```python
from build123d import *

# Parameters (mm, degrees)
EXTRUDE_1_DEPTH     = 3
FILLET_1_R          = 6
FILLET_2_R          = 2
SKETCH_2_R          = 1.65
CUT_EXTRUDE_1_DEPTH = 5
FILLET_3_R          = 10
SKETCH_3_W          = 90
SKETCH_3_H          = 4
CUT_EXTRUDE_2_DEPTH = 10
FILLET_4_R          = 10


with BuildPart() as part:
    # 草图1 → 凸台-拉伸1 (new body)
    with BuildSketch(Plane.XY):
        Polygon((25, 25), (45, 25), (45, -25), (-45, -25), (-45, 25), (-25, 25), (-25, 20), (-36, 20), (-36, 5), (36, 5), (36, 20), (25, 20), align=None)
    extrude(amount=EXTRUDE_1_DEPTH)

    # 圆角1
    fillet_1_edges = [part.edges().sort_by_distance(p)[0] for p in [
        (-45, 25, 1.5),
        (45, 25, 1.5),
    ]]
    fillet(fillet_1_edges, radius=FILLET_1_R)

    # 圆角2
    fillet_2_edges = [part.edges().sort_by_distance(p)[0] for p in [
        (-25, 25, 1.5),
        (-25, 20, 1.5),
        (-36, 20, 1.5),
        (-36, 5, 1.5),
        (36, 5, 1.5),
        (36, 20, 1.5),
        (25, 20, 1.5),
        (25, 25, 1.5),
    ]]
    fillet(fillet_2_edges, radius=FILLET_2_R)

    # 草图2 → 切除-拉伸1 (cut)
    with BuildSketch(Plane.XY.offset(3)):
        with Locations((-25, -10)):
            Circle(SKETCH_2_R)
        with Locations((25, -10)):
            Circle(SKETCH_2_R)
        with Locations((0, -10)):
            Circle(SKETCH_2_R)
    extrude(amount=-CUT_EXTRUDE_1_DEPTH, mode=Mode.SUBTRACT)

    # 圆角3
    fillet_3_edges = [part.edges().sort_by_distance(p)[0] for p in [
        (45, -25, 1.5),
        (-45, -25, 1.5),
    ]]
    fillet(fillet_3_edges, radius=FILLET_3_R)

    # 草图3 → 切除-拉伸2 (cut)
    with BuildSketch(Plane.XY.offset(3)):
        with Locations((0, -23)):
            Rectangle(SKETCH_3_W, SKETCH_3_H)
    extrude(amount=-CUT_EXTRUDE_2_DEPTH, mode=Mode.SUBTRACT)

    # 圆角4
    fillet_4_edges = [part.edges().sort_by_distance(p)[0] for p in [
        (43, -21, 1.5),
    ]]
    fillet(fillet_4_edges, radius=FILLET_4_R)
    fillet_4_2_edges = [part.edges().sort_by_distance(p)[0] for p in [
        (-43, -21, 1.5),
    ]]
    fillet(fillet_4_2_edges, radius=FILLET_4_R)


solid = part.part
```
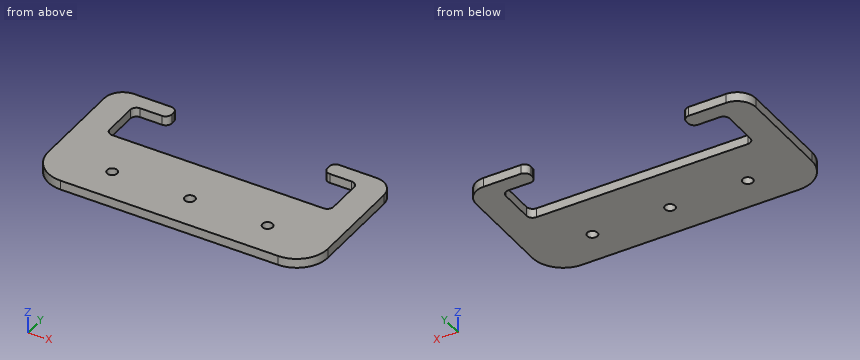
For this review, take the finished solid that the model builds, in its own axes (mm). Round coordinates to 2 decimals unless told otherwise and drop trailing zeros. Write each loop counter-clockwise with the first axis right and the second up, starting at its lowest first coordinate (ties: lowest second). Pieces come first, ordered by that corner, then holes. Notation, with made-up numbers: M 30.25,78 L 87.25,78 A34 ccw 87.25,111 Z; hole C 86.5,27.5 d6. An arc over 180 degrees is marked long. One line per item, written item: value. Start each with the question number.
(1) Wall thickness on line 1 (Y direction, x = 0, z = 2.15); line 2 (X direction, y = 7, z = 2.05); line 3 (Y direction, x = -29.5, z = 2.15): over which ranges is each line inside the solid? List them lowest first.
(2) We need section C-C (y = 10). Give the boundary of the cut face in (x, z), and give its area (3 significant figures).
(3) We need section D-D (z = 1.85). Count the separate pieces of the cut face and the enclosed holes in it, and give its area (3 significant figures).
(4) Insertion check: pin 1 (0.8 mm diameter, centred on y = 22.5, z = 1, fed in from +X); pin 2 (0.8 mm diameter, centred on y = 22.5, z = 1.5, fed in from -X); pin 3 (0.9 mm diameter, centred on x = -6, z = 1.5, fed in from +Y). Each pin has a flat end and moves straight along its axis. Give the tip position at first contact, or say it passes through.
(5) We need section B-B (x = 0). Give the boundary of the cut face in (y, z).
(6) We need section A-A (y = -10). Give the boundary of the cut face in (x, z).
Result:
1. line 1: -21 to -11.65, -8.35 to 5
1. line 2: -45 to -36, 36 to 45
1. line 3: -21 to 5, 20 to 25
2. outline: M -45,0 L -36,0 L -36,3 L -45,3 Z; M 36,0 L 45,0 L 45,3 L 36,3 Z
2. area: 54.0 mm²
3. separate pieces: 1
3. enclosed holes: 3
3. area: 2,730 mm²
4. pin 1: x = 44.14
4. pin 2: x = -44.14
4. pin 3: y = 5
5. outline: M -21,0 L -11.65,0 L -11.65,3 L -21,3 Z; M -8.35,0 L 5,0 L 5,3 L -8.35,3 Z
6. outline: M -45,0 L -26.65,0 L -26.65,3 L -45,3 Z; M -23.35,0 L -1.65,0 L -1.65,3 L -23.35,3 Z; M 1.65,0 L 23.35,0 L 23.35,3 L 1.65,3 Z; M 26.65,0 L 45,0 L 45,3 L 26.65,3 Z
